Can you work these out from the model? Positions are in its coordinate system, mm. Give positions to 0.01 mm unless a question says otherwise; leave off trailing zeros. Write each loop counter-clockwise with the first axis right and the second up, starting at its lowest first coordinate (ties: lowest second). Pieces come first, ordered by that corner, then holes.
1. I'm going to push a flat-ended pin straight in: pin 1 (8 mm diameter, centred on x = 2, y = 9.5, fed in from -Z). Where does the tip first touch, or does it pass through?
2. Suppose I cut it at C-C (y = 6.5). Please give me the cut outline in (x, z) (3 decimals), and give its area (3 significant figures).
3. Suppose I cut it at A-A (x = 0). Please give me the cut outline in (y, z) (3 decimals), and give its area (3 significant figures).
4. Suppose I cut it at B-B (y = 12.7). Please give me the cut outline in (x, z) (3 decimals).
5. Suppose I cut it at D-D (x = 4.75). Please give me the cut outline in (y, z) (3 decimals).
6. If I drill on probe 1 along Z at (x, y) = (3.75, 1.5), over which ranges is the centre line in solid material (lowest first)?
```python
from build123d import *

# Parameters (mm, degrees)
SKETCH001_R  = 0.35
PAD001_DEPTH = 3.5
SKETCH_W     = 16.13
SKETCH_H     = 16.13
PAD_DEPTH    = 9.27
FILLET_R     = 0.7


with BuildPart() as pad001:
    # Sketch001 → Pad001 (new body)
    with BuildSketch(Plane.XY.offset(0.5)):
        Circle(SKETCH001_R)
        with Locations((7.62, 12.7)):
            Circle(SKETCH001_R)
    extrude(amount=-PAD001_DEPTH)


with BuildPart() as obj1:
    # Sketch → Pad (new body)
    with BuildSketch(Plane.XY.offset(0.1)):
        with Locations((3.81, 6.35)):
            Rectangle(SKETCH_W, SKETCH_H)
    extrude(amount=PAD_DEPTH)

    # Fillet
    fillet_edges = [obj1.edges().sort_by_distance(p)[0] for p in [
        (11.875, -1.715, 4.735),
        (11.875, 14.415, 4.735),
        (-4.255, -1.715, 4.735),
        (-4.255, 14.415, 4.735),
    ]]
    fillet(fillet_edges, radius=FILLET_R)

    # obj1: union Pad001
    add(pad001.part)


solid = obj1.part
```
Checks:
1. pin 1: stops at z = 0.1
2. outline: (-4.255, 0.1) - (11.875, 0.1) - (11.875, 9.37) - (-4.255, 9.37) - close
2. area: 150 mm2
3. outline: (-1.715, 0.1) - (-0.35, 0.1) - (-0.35, -3) - (0.35, -3) - (0.35, 0.1) - (14.415, 0.1) - (14.415, 9.37) - (-1.715, 9.37) - close
3. area: 152 mm2
4. outline: (-4.255, 0.1) - (7.27, 0.1) - (7.27, -3) - (7.97, -3) - (7.97, 0.1) - (11.875, 0.1) - (11.875, 9.37) - (-4.255, 9.37) - close
5. outline: (-1.715, 0.1) - (14.415, 0.1) - (14.415, 9.37) - (-1.715, 9.37) - close
6. probe 1: z = 0.1 to 9.37
